For this review, use the dimensioned drawing (mm, ordinates from the lowest corner) and the shaded views. Give positions to 0.01 mm unless a question says otherwise; leave off trailing zeros. Write each loop counter-clockwise with the first axis right and the second up, starting at its lowest first coordinate (ties: lowest second). Pieces come first, ordered by that corner, then holes. Notation, with made-up numbers: (-0.5, 35.25) -> (16.5, 35.25) arc R21 cw to (16.5, 48.25) -> close; hole circle Ø6 at (10.25, 66). An arc over 180 degrees is marked (long way). Answer as CSV lines item,"result".
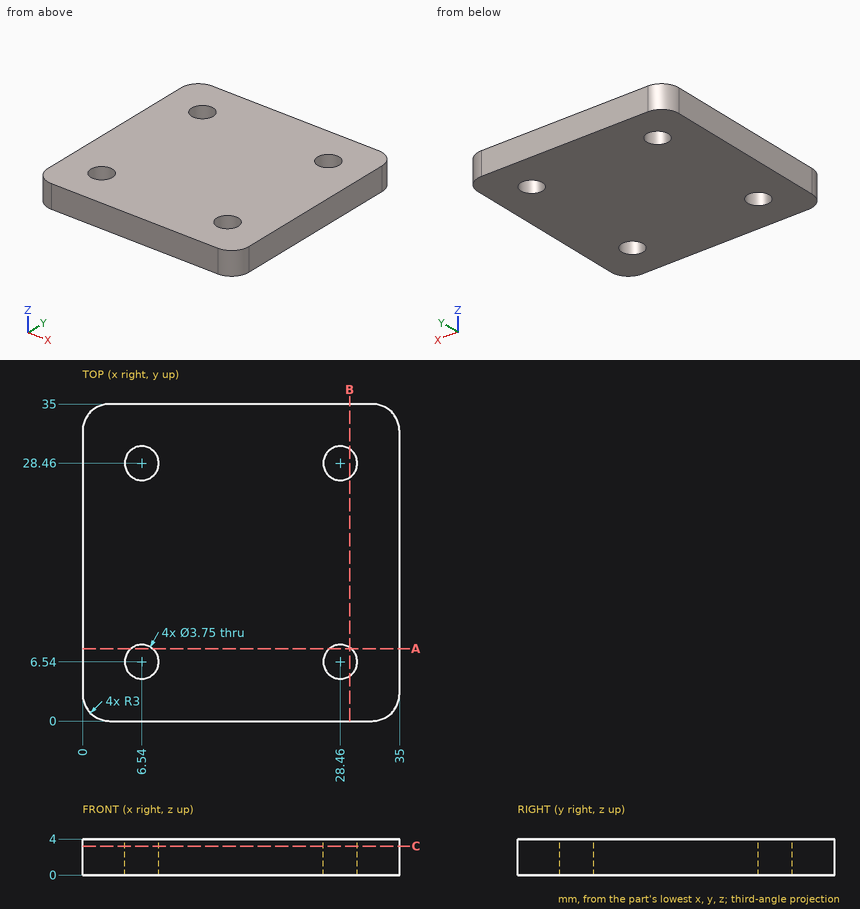
Q1. Clearance check with a flat-ended pin moving along its axis: pin 1 (2 mm diameter, centred on x = 28.46, y = 6.54, fed in from -Z). State where the tip first meets the part, or that it passes through.
Answer block:
pin 1,"passes through"
Q2. To check wall thickness, follow probe 1 along Y at (x, z) = (28.5, 1) (1 decimal); probe 2 along Y at (x, z) = (27.5, 3.8); probe 3 along X at (y, z) = (28, 3.7). State the ranges of each line that lie inside material, in increasing order. Write a range as [from, to].
Answer block:
probe 1,"y = [0, 4.7], [8.4, 26.6], [30.3, 35]"
probe 2,"y = [0, 4.93], [8.15, 26.85], [30.07, 35]"
probe 3,"x = [0, 4.72], [8.36, 26.64], [30.28, 35]"
Q3. Add section B-B (x = 29.5). Write out the cut boundary in (y, z).
Answer block:
outline,"(0, 0) -> (4.98, 0) -> (4.98, 4) -> (0, 4) -> close; (8.1, 0) -> (26.9, 0) -> (26.9, 4) -> (8.1, 4) -> close; (30.02, 0) -> (35, 0) -> (35, 4) -> (30.02, 4) -> close"
Q4. Add section A-A (y = 8). Write out the cut boundary in (x, z), plus the area to 3 significant figures.
Answer block:
outline,"(0, 0) -> (5.36, 0) -> (5.36, 4) -> (0, 4) -> close; (7.72, 0) -> (27.28, 0) -> (27.28, 4) -> (7.72, 4) -> close; (29.64, 0) -> (35, 0) -> (35, 4) -> (29.64, 4) -> close"
area,"121 mm2"
Q5. Add section C-C (z = 3.2). Write out the cut boundary in (x, y) (3 decimals).
Answer block:
outline,"(0, 3) arc R3 ccw to (3, 0) -> (32, 0) arc R3 ccw to (35, 3) -> (35, 32) arc R3 ccw to (32, 35) -> (3, 35) arc R3 ccw to (0, 32) -> close; hole circle Ø3.75 at (6.54, 6.54); hole circle Ø3.75 at (6.54, 28.46); hole circle Ø3.75 at (28.46, 6.54); hole circle Ø3.75 at (28.46, 28.46)"
